from build123d import *

# Parameters (mm, degrees)
EXTRUDE_1_DEPTH             = 18
CUT_EXTRUDE_1_DEPTH         = 15
EXTRUDE_2_DEPTH             = 15
HOLE_WIZARD_4_5_4_5_1_D     = 4.5
HOLE_WIZARD_4_5_4_5_1_DEPTH = 18
HOLE_WIZARD_10_0_10_1_D     = 10
HOLE_WIZARD_10_0_10_1_DEPTH = 18
HOLE_WIZARD_15_0_15_1_D     = 15
HOLE_WIZARD_15_0_15_1_DEPTH = 18
FILLET_1_R                  = 1


with BuildPart() as part:
    # 草图1 → 凸台-拉伸1 (new body)
    with BuildSketch(Plane(origin=(0, 0, 0), x_dir=(-1, 0, 0), z_dir=(0, 0, -1))):
        with BuildLine():
            ThreePointArc((-63.022889612, -268.325738264), (-50, -366.6), (-36.977110388, -268.325738264))
            ThreePointArc((-36.977110388, -268.325738264), (-41.171867667, -269.55111981), (-45.000340281, -271.658332659))
            ThreePointArc((-45.000340281, -271.658332659), (-50, -266.6), (-54.999659719, -271.658332659))
            ThreePointArc((-54.999659719, -271.658332659), (-58.828132333, -269.55111981), (-63.022889612, -268.325738264))
        make_face()
    extrude(amount=-EXTRUDE_1_DEPTH)

    # 草图2 → 切除-拉伸1 (cut)
    with BuildSketch(Plane.XY.offset(18)):
        with BuildLine():
            Line((76.956193034, -333.068180736), (77.765412233, -331.666571969))
            ThreePointArc((77.765412233, -331.666571969), (97.88324923, -322.335101774), (89.229210711, -301.916695402))
            ThreePointArc((89.229210711, -301.916695402), (88.637121061, -301.181657), (88.92041407, -300.281325574))
            ThreePointArc((88.92041407, -300.281325574), (89.825644155, -293.580135017), (83.548411657, -291.065826255))
            ThreePointArc((83.548411657, -291.065826255), (82.62171892, -290.865593126), (82.278658267, -289.981759362))
            ThreePointArc((82.278658267, -289.981759362), (69.366720715, -272.381727147), (51.051780987, -284.257848066))
            ThreePointArc((51.051780987, -284.257848066), (50.716834815, -284.792322878), (50.128600006, -285.01998946))
            ThreePointArc((50.128600006, -285.01998946), (49.538997539, -284.791191751), (49.204585003, -284.254397827))
            ThreePointArc((49.204585003, -284.254397827), (30.663154881, -272.122268325), (17.461812053, -289.918271942))
            ThreePointArc((17.461812053, -289.918271942), (17.131459448, -290.784603767), (16.231387053, -291.007164675))
            ThreePointArc((16.231387053, -291.007164675), (10.151561622, -293.619612904), (10.9830551, -300.184502973))
            ThreePointArc((10.9830551, -300.184502973), (11.246762281, -301.077699779), (10.659953012, -301.80088502))
            ThreePointArc((10.659953012, -301.80088502), (1.85480976, -322.061978817), (21.565140626, -332.039219251))
            ThreePointArc((21.565140626, -332.039219251), (22.17257693, -332.052081262), (22.660452123, -332.414189106))
            ThreePointArc((22.660452123, -332.414189106), (22.73017699, -333.017409123), (22.438041219, -333.549755475))
            ThreePointArc((22.438041219, -333.549755475), (21.244961438, -355.543032932), (43.131077631, -358.018030031))
            ThreePointArc((43.131077631, -358.018030031), (44.05505938, -357.871893349), (44.695584039, -358.553675105))
            ThreePointArc((44.695584039, -358.553675105), (50.022786366, -362.599952798), (55.316278846, -358.509673449))
            ThreePointArc((55.316278846, -358.509673449), (55.955599054, -357.821048903), (56.883882353, -357.966734219))
            ThreePointArc((56.883882353, -357.966734219), (78.956360747, -355.220704534), (76.956193034, -333.068180736))
        make_face()
    extrude(amount=-CUT_EXTRUDE_1_DEPTH, mode=Mode.SUBTRACT)

    # 草图3 → 凸台-拉伸2 (add)
    with BuildSketch(Plane.XY.offset(3)):
        with BuildLine():
            Line((71.709131996, -303.043642956), (72.56925981, -304.533428031))
            ThreePointArc((72.56925981, -304.533428031), (67.05, -316.6), (72.56925981, -328.666571969))
            Line((72.56925981, -328.666571969), (71.760040611, -330.068180736))
            ThreePointArc((71.760040611, -330.068180736), (58.841180082, -331.130974521), (50.949212572, -341.414132443))
            ThreePointArc((50.949212572, -341.414132443), (50.614490777, -341.949534813), (50.02571996, -342.177664826))
            ThreePointArc((50.02571996, -342.177664826), (49.436675631, -341.949308595), (49.102060561, -341.41344243))
            ThreePointArc((49.102060561, -341.41344243), (41.525, -331.279130594), (28.959898219, -329.78435958))
            ThreePointArc((28.959898219, -329.78435958), (28.35280487, -329.771183403), (27.865263445, -329.409189888))
            ThreePointArc((27.865263445, -329.409189888), (27.79560645, -328.805623655), (28.088185773, -328.273137379))
            ThreePointArc((28.088185773, -328.273137379), (33.1, -316.6), (28.088185773, -304.926862621))
            ThreePointArc((28.088185773, -304.926862621), (27.800926844, -304.419745345), (27.845189576, -303.838602992))
            ThreePointArc((27.845189576, -303.838602992), (28.326676887, -303.509594278), (28.909820681, -303.505113168))
            ThreePointArc((28.909820681, -303.505113168), (41.575, -302.007471946), (49.204585003, -291.787925524))
            ThreePointArc((49.204585003, -291.787925524), (49.538997539, -291.251131599), (50.128600006, -291.02233389))
            ThreePointArc((50.128600006, -291.02233389), (50.716834815, -291.250000473), (51.051780987, -291.784475285))
            ThreePointArc((51.051780987, -291.784475285), (58.890667579, -301.982109354), (71.709131996, -303.043642956))
        make_face()
    extrude(amount=EXTRUDE_2_DEPTH)

    # Ø4.5 (4.5) 直径孔1
    with Locations(Plane.XY.offset(18)):
        with Locations((50, -271.6)):
            Hole(HOLE_WIZARD_4_5_4_5_1_D / 2, depth=HOLE_WIZARD_4_5_4_5_1_DEPTH)

    # Ø10.0 (10) 直径孔1
    with Locations(Plane.XY.offset(18)):
        with Locations((50, -316.6)):
            Hole(HOLE_WIZARD_10_0_10_1_D / 2, depth=HOLE_WIZARD_10_0_10_1_DEPTH)

    # Ø15.0 (15) 直径孔1
    with Locations(Plane(origin=(0, 0, 0), x_dir=(-1, 0, 0), z_dir=(0, 0, -1))):
        with Locations((-33.5, -288.021161675), (-83, -316.6), (-66.5, -345.178838325), (-33.5, -345.178838325), (-66.5, -288.021161675), (-17, -316.6)):
            Hole(HOLE_WIZARD_15_0_15_1_D / 2, depth=HOLE_WIZARD_15_0_15_1_DEPTH)

    # 圆角1
    fillet_1_edges = [part.edges().sort_by_distance(p)[0] for p in [
        (77.765412233, -331.666571969, 10.5),
        (76.956193034, -333.068180736, 10.5),
        (71.760040611, -330.068180736, 10.5),
        (72.56925981, -328.666571969, 10.5),
        (72.56925981, -304.533428031, 10.5),
        (71.709131996, -303.043642956, 10.5),
    ]]
    fillet(fillet_1_edges, radius=FILLET_1_R)


solid = part.part
The listing builds one solid part. Answer for the finished solid, in the listing's coordinates (mm). A direction names the side the tool comes from. Coordinates: 2 decimals unless noted, no trailing zeros. Write each loop counter-clockwise with the first axis right and the second up, starting at its lowest first coordinate (ties: lowest second). Pieces come first, ordered by that corner, then holes. Notation, with made-up numbers: M 1,-24.75 L 23,-24.75 A12 cw 23,-2.75 Z; hole C -39,-1 d6. An arc over 180 degrees is marked long. Put each result on its own line as item: value. Start each with the question number.
1. Which of the six approach directions +Z, -Z, +X, -X, +Y, -Y give full straight-line access (tool end or side, diameter ignored) to faces 1 (the flat face through (50, -283, 18)), 2 (the cylindrical face through (78.485, -355.778, 10.605))?
2. Consider line 1 (X direction, y = -316.6, z = 1.1); line 2 (Y direction, x = 50, z = 14.25); line 3 (X direction, y = -337, z = 15.5). Determine where each line is inside the solid, lowest interval first. Write a range as from..to.
3. A cutting plane is placed at A-A on y = -325.5. Write down the section's boundary in (x, z), then the cut area to 3 significant figures.
4. A cutting plane is placed at C-C on z = 13.75. Count the separate pieces of the cut face and the enclosed holes in it, then the cut area to 3 significant figures.
5. For a pull along X with two mould halves and no side action, classify faces 3 (the cylindrical face through (52.01, -366.56, 8.87)), 4 (the flat face through (55.3, -316.2, 18)), 5 (the cylindrical face through (49.9, -266.6, 8.9)) as pulls with the +X half, pulls with the -X half, needs draft (parallel to the pull), parting line crosses it, or undercut.
6. Flat-ended cylindrical pins translate along their axes: P1, Ø2, axis at x = 46.5, z = 13, coming from the -Y side; P2, Ø10, axis at y = -339.5, z = 10, coming from the -X side; P3, Ø5, axis at y = -287, z = 8, coming from the +X side. Find the tip coordinate at first contact, or state that the pin passes through.
7. A cutting plane is placed at D-D on x = 8. Write down the section's boundary in (y, z).
8. A cutting plane is placed at B-B on x = 93. Write down the section's boundary in (y, z).
Resolved:
1. face 1: +Z, +X, -X, +Y, -Y
1. face 2: +Z
2. line 1: x = 0..9.5, 24.5..45, 55..75.5, 90.5..100
2. line 2: y = -366.6..-362.6, -342.18..-321.6, -311.6..-291.04, -285.01..-273.85, -269.35..-266.6
2. line 3: x = 4.35..19.69, 47.31..52.75, 80.25..95.65
3. outline: M 0.8,0 L 99.2,0 L 99.2,18 L 96.24,18 L 96.24,3 L 69.76,3 L 69.76,18 L 30.42,18 L 30.42,3 L 3.58,3 L 3.58,18 L 0.8,18 Z
3. area: 972 mm2
4. separate pieces: 2
4. enclosed holes: 3
4. area: 2,540 mm2
5. face 3: parting line crosses it
5. face 4: needs draft
5. face 5: undercut
6. P1: stops at y = -366.54
6. P2: stops at x = 3.31
6. P3: stops at x = 92.02
7. outline: M -343.73,0 L -289.47,0 L -289.47,18 L -303.25,18 L -303.25,3 L -329.95,3 L -329.95,18 L -343.73,18 Z
8. outline: M -342.11,0 L -291.09,0 L -291.09,18 L -304.17,18 L -304.17,3 L -329.03,3 L -329.03,18 L -342.11,18 Z
